Geometry: final body of the model. Coordinates: model frame, mm. A direction names the side the tool comes from. Coordinates: 2 decimals unless noted, no trailing zeros. Order: outer loops, then holes, each group sorted by start corner. A loop starts at its lowest first (then second) coordinate and runs counter-clockwise, first axis right, second up. Notation, with made-up numbers: M 66.5,31 L 75.5,31 A20 cw 75.5,36 Z; hole C 17.5,86.25 d4. An arc over 180 degrees is marked long. Use CSV: the item, a comma, the result in double quotes. Start each with the question number.
Q1. Ray query, probe 1 along Y at (x, z) = (-17, 57); probe 2 along Z at (x, y) = (0, 9); probe 3 along Z at (x, y) = (0, 72). Return the intervals inside material, ascending.
Q2. Section query D-D, the plane z = 74. Output: boundary loops of the cut face in (x, y).
Q3. Section query A-A, the plane x = 0. Output: boundary loops of the cut face in (y, z), and give its area (3 significant figures).
Q4. Mould query, pull axis Y, two halves, no side actions, for faces 6 (the face through (8.44, 62.61, -16.23)), 7 (the face through (18.294, 114, 34)), 8 (the face through (0, 0, 36)). Classes: +Y half, -Y half, draft (parallel to the pull), parting line (faces both ways), or undercut.
Q5. First-contact query: P1, Ø7.5, axis at y = 8, z = 39, coming from the -X side; P2, Ø5, axis at x = 3, y = 109.5, coming from the -Z side; P3, Ø12.5, axis at x = 0, z = 70.88, coming from the +Y side; P4, Ø12.5, axis at y = 114.5, z = 21, coming from the +X side. Flat tips, straight axial feed; report the tip coordinate or a pass-through.
Q6. Section query C-C, the plane y = 82.5. Output: boundary loops of the cut face in (x, z), and give its area (3 significant figures).
Q7. Access query for faces 1 (the face through (-8.192, 62.611, -6.282)), 2 (the face through (18.294, 13, 33)), 3 (the face through (-18.294, 114, 33)), 4 (the face through (0, 127, 36)), 5 (the face through (-1.34, 12.52, 80.99)). Directions: +Z, -Z, +X, -X, +Y, -Y. A direction counts if a zero-diameter tool reaches every point of the face in a straight line with its end or side. Return the directions, or none.
Q8. Section query B-B, the plane z = 59. Output: boundary loops of the cut face in (x, y), and give its area (3 significant figures).
from build123d import *

# Parameters (mm, degrees)
F0_R     = 10.323224
F1_DEPTH = 127
F2_DEPTH = 25.4
F3_R     = 10.223402
F4_DEPTH = 25.4


with BuildPart() as f1:
    # F0 (on Front) → F1 (new body)
    with BuildSketch(Plane.XZ):
        with BuildLine():
            ThreePointArc((-18.294126, 0), (0, -18.294126), (18.294126, 0))
            ThreePointArc((18.294126, 0), (0, 18.294126), (-18.294126, 0))
        make_face()
        Circle(F0_R, mode=Mode.SUBTRACT)
    extrude(amount=-F1_DEPTH)

    # F0 (on Front) → F2 (join)
    with BuildSketch(Plane.XZ):
        with BuildLine():
            ThreePointArc((-18.294126, 0), (0, -18.294126), (18.294126, 0))
            ThreePointArc((18.294126, 0), (0, 18.294126), (-18.294126, 0))
        make_face()
        Circle(F0_R, mode=Mode.SUBTRACT)
        with BuildLine():
            ThreePointArc((-18.294126, 0), (0, 18.294126), (18.294126, 0))
            Line((18.294126, 0), (18.294126, 67.357816))
            ThreePointArc((18.294126, 67.357816), (0, 89.361622), (-18.294126, 67.357816))
            Line((-18.294126, 67.357816), (-18.294126, 0))
        make_face()
        with Locations((0, 70.754784)):
            Circle(F0_R, mode=Mode.SUBTRACT)
    extrude(amount=-F2_DEPTH)

    # F3 (on face) → F4 (join)
    with BuildSketch(Plane(origin=(0, 127, 0), x_dir=(-1, 0, 0), z_dir=(0, 1, 0))):
        with BuildLine():
            Line((-18.294126, 67.450888), (-18.294126, 0))
            ThreePointArc((-18.294126, 0), (0, 18.294126), (18.294126, 0))
            Line((18.294126, 0), (18.294126, 67.450888))
            ThreePointArc((18.294126, 67.450888), (0, 89.491754), (-18.294126, 67.450888))
        make_face()
        with Locations((0, 70.879173)):
            Circle(F3_R, mode=Mode.SUBTRACT)
    extrude(amount=-F4_DEPTH)


solid = f1.part
Responses:
1,probe 1,"y = 0 to 25.4, 101.6 to 127"
1,probe 2,"z = -18.29 to -10.32, 10.32 to 60.43, 81.08 to 89.36"
1,probe 3,"z = -18.29 to -10.32, 10.32 to 18.29"
2,outline,"M -18.35,101.6 L -9.74,101.6 L -9.74,127 L -18.35,127 Z; M -18.32,0 L -9.8,0 L -9.8,25.4 L -18.32,25.4 Z; M 9.74,101.6 L 18.35,101.6 L 18.35,127 L 9.74,127 Z; M 9.8,0 L 18.32,0 L 18.32,25.4 L 9.8,25.4 Z"
3,outline,"M 0,-18.29 L 127,-18.29 L 127,-10.32 L 0,-10.32 Z; M 0,10.32 L 127,10.32 L 127,60.66 L 101.6,60.66 L 101.6,18.29 L 25.4,18.29 L 25.4,60.43 L 0,60.43 Z; M 0,81.08 L 25.4,81.08 L 25.4,89.36 L 0,89.36 Z; M 101.6,81.1 L 127,81.1 L 127,89.49 L 101.6,89.49 Z"
3,area,"4,590 mm²"
4,face 6,"undercut"
4,face 7,"draft"
4,face 8,"-Y half"
5,P1,"stops at x = -18.29"
5,P2,"stops at z = -18.29"
5,P3,"passes through"
5,P4,"stops at x = 18.29"
6,outline,"C 0,0 d36.59; hole C 0,0 d20.65"
6,area,"717 mm²"
7,face 1,"+Y, -Y"
7,face 2,"-Z, +X, +Y, -Y"
7,face 3,"-Z, -X, +Y, -Y"
7,face 4,"+Z, -Z, +X, -X, +Y"
7,face 5,"-Y"
8,outline,"M -18.29,0 L 18.29,0 L 18.29,25.4 L -18.29,25.4 Z; M -18.29,101.6 L 18.29,101.6 L 18.29,127 L -18.29,127 Z"
8,area,"1,860 mm²"
